Input: part model. Units: mm. Frame: model coordinates. Round coordinates to 2 decimals unless told otherwise and drop trailing zeros. Order: outer loops, then holes, each group sorted by start corner. A loop starts at its lowest first (then second) coordinate and runs counter-clockwise, first axis right, second up. Notation, with made-up numbers: (71.5, 81.5) -> (109.5, 81.5) arc R25 cw to (109.5, 93.5) -> close; hole circle Ø2 at (-19, 79.5). An arc over 180 degrees is marked (long way). Answer as CSV lines item,"result". Start each with the question number.
1) First-contact query: P1, Ø1.4, axis at x = -253.5, z = 2, coming from the +Y side. Flat tip, straight axial feed; report the tip coordinate or a pass-through.
2) Mould query, pull axis Y, two halves, no side actions, for faces 1 (the face through (-220, 38, 0)), 2 (the face through (-4.63, 89.34, 2.35)), 3 (the face through (-208.424, 10.662, 2.348)). Classes: +Y half, -Y half, draft (parallel to the pull), parting line (faces both ways), or undercut.
3) Section query B-B, the plane z = 3.45. State how many separate pieces and enclosed holes the cut face has, and give its area (3 significant figures).
4) Line query: L1, parallel to X at y = 18, z = 1.8; L2, parallel to X at y = 6, z = 0.75; L3, parallel to Y at x = -363, z = 3.3. Output: solid intervals per line, ascending.
5) Section query A-A, the plane y = 4. Output: boundary loops of the cut face in (x, z), and give its area (3 significant figures).
```python
from build123d import *

# Parameters (mm, degrees)
SKETCH1_R           = 14.225
SKETCH1_R_2         = 14.3
SKETCH1_R_3         = 3.18
SKETCH1_R_4         = 1.25
BOSS_EXTRUDE5_DEPTH = 4.7625


with BuildPart() as part:
    # Sketch1 → Boss-Extrude5 (new body)
    with BuildSketch(Plane.XY):
        with BuildLine():
            Line((-438.54516333, 90.490429708), (-13.66516333, 90.490429708))
            ThreePointArc((-13.66516333, 90.490429708), (-4.523203097, 89.26845658), (-0.269770336, 81.084511017))
            Line((-0.269770336, 81.084511017), (-0.269770336, -5.909570292))
            ThreePointArc((-0.269770336, -5.909570292), (-3.198702525, -12.980638104), (-10.269770336, -15.909570292))
            Line((-10.269770336, -15.909570292), (-435.149770336, -15.909570292))
            ThreePointArc((-435.149770336, -15.909570292), (-442.220838148, -12.980638104), (-445.149770336, -5.909570292))
            Line((-445.149770336, -5.909570292), (-445.149770336, 81.084511017))
            ThreePointArc((-445.149770336, 81.084511017), (-443.333715899, 86.831078256), (-438.54516333, 90.490429708))
        make_face()
        with Locations(Location((-394.349770336, 12.790429708, 0), (0, 0, 180))):
            Circle(SKETCH1_R, mode=Mode.SUBTRACT)
        with Locations(Location((-51.069770336, 12.790429708, 0), (0, 0, 180))):
            Circle(SKETCH1_R, mode=Mode.SUBTRACT)
        with Locations(Location((-222.709770336, 11.290429708, 0), (0, 0, 180))):
            Circle(SKETCH1_R_2, mode=Mode.SUBTRACT)
        with Locations(Location((-174.899770336, 13.384511017, 0), (0, 0, 180))):
            Circle(SKETCH1_R_3, mode=Mode.SUBTRACT)
        with Locations(Location((-366.990768764, 12.790429708, 0), (0, 0, 180))):
            Circle(SKETCH1_R_3, mode=Mode.SUBTRACT)
        with Locations(Location((-358.995687615, 21.719099167, 0), (0, 0, 180))):
            Circle(SKETCH1_R_4, mode=Mode.SUBTRACT)
        with Locations(Location((-94.899770336, 13.384511017, 0), (0, 0, 180))):
            Circle(SKETCH1_R_3, mode=Mode.SUBTRACT)
        with Locations(Location((-96.899770336, 21.384511017, 0), (0, 0, 180))):
            Circle(SKETCH1_R_4, mode=Mode.SUBTRACT)
        with Locations(Location((-106.899770336, 21.384511017, 0), (0, 0, 180))):
            Circle(SKETCH1_R_4, mode=Mode.SUBTRACT)
        with Locations(Location((-350.990768764, 12.790429708, 0), (0, 0, 180))):
            Circle(SKETCH1_R_3, mode=Mode.SUBTRACT)
        with Locations(Location((-334.990768764, 12.790429708, 0), (0, 0, 180))):
            Circle(SKETCH1_R_3, mode=Mode.SUBTRACT)
        with Locations(Location((-318.990768764, 12.790429708, 0), (0, 0, 180))):
            Circle(SKETCH1_R_3, mode=Mode.SUBTRACT)
        with Locations(Location((-302.990768764, 12.790429708, 0), (0, 0, 180))):
            Circle(SKETCH1_R_3, mode=Mode.SUBTRACT)
        with Locations(Location((-286.990768764, 12.790429708, 0), (0, 0, 180))):
            Circle(SKETCH1_R_3, mode=Mode.SUBTRACT)
        with Locations(Location((-158.899770336, 13.384511017, 0), (0, 0, 180))):
            Circle(SKETCH1_R_3, mode=Mode.SUBTRACT)
        with Locations(Location((-142.899770336, 13.384511017, 0), (0, 0, 180))):
            Circle(SKETCH1_R_3, mode=Mode.SUBTRACT)
        with Locations(Location((-126.899770336, 13.384511017, 0), (0, 0, 180))):
            Circle(SKETCH1_R_3, mode=Mode.SUBTRACT)
        with Locations(Location((-110.899770336, 13.384511017, 0), (0, 0, 180))):
            Circle(SKETCH1_R_3, mode=Mode.SUBTRACT)
        with Locations(Location((-86.899770336, 21.384511017, 0), (0, 0, 180))):
            Circle(SKETCH1_R_4, mode=Mode.SUBTRACT)
        with Locations(Location((-270.990768764, 12.790429708, 0), (0, 0, 180))):
            Circle(SKETCH1_R_3, mode=Mode.SUBTRACT)
        with Locations(Location((-348.995687615, 21.719099167, 0), (0, 0, 180))):
            Circle(SKETCH1_R_4, mode=Mode.SUBTRACT)
        with Locations(Location((-116.899770336, 21.384511017, 0), (0, 0, 180))):
            Circle(SKETCH1_R_4, mode=Mode.SUBTRACT)
        with Locations(Location((-338.995687615, 21.719099167, 0), (0, 0, 180))):
            Circle(SKETCH1_R_4, mode=Mode.SUBTRACT)
        with Locations(Location((-328.995687615, 21.719099167, 0), (0, 0, 180))):
            Circle(SKETCH1_R_4, mode=Mode.SUBTRACT)
        with Locations(Location((-318.995687615, 21.719099167, 0), (0, 0, 180))):
            Circle(SKETCH1_R_4, mode=Mode.SUBTRACT)
        with Locations(Location((-308.995687615, 21.719099167, 0), (0, 0, 180))):
            Circle(SKETCH1_R_4, mode=Mode.SUBTRACT)
        with Locations(Location((-298.995687615, 21.719099167, 0), (0, 0, 180))):
            Circle(SKETCH1_R_4, mode=Mode.SUBTRACT)
        with Locations(Location((-288.995687615, 21.719099167, 0), (0, 0, 180))):
            Circle(SKETCH1_R_4, mode=Mode.SUBTRACT)
        with Locations(Location((-126.899770336, 21.384511017, 0), (0, 0, 180))):
            Circle(SKETCH1_R_4, mode=Mode.SUBTRACT)
        with Locations(Location((-136.899770336, 21.384511017, 0), (0, 0, 180))):
            Circle(SKETCH1_R_4, mode=Mode.SUBTRACT)
        with Locations(Location((-146.899770336, 21.384511017, 0), (0, 0, 180))):
            Circle(SKETCH1_R_4, mode=Mode.SUBTRACT)
        with Locations(Location((-156.899770336, 21.384511017, 0), (0, 0, 180))):
            Circle(SKETCH1_R_4, mode=Mode.SUBTRACT)
        with Locations(Location((-222.709770336, 85.384511017, 0), (0, 0, 180))):
            Circle(SKETCH1_R_4, mode=Mode.SUBTRACT)
        with Locations(Location((-142.709770336, 78.334511017, 0), (0, 0, 180))):
            Circle(SKETCH1_R_3, mode=Mode.SUBTRACT)
        with Locations(Location((-94.709770336, 78.334511017, 0), (0, 0, 180))):
            Circle(SKETCH1_R_3, mode=Mode.SUBTRACT)
        with Locations(Location((-78.709770336, 78.334511017, 0), (0, 0, 180))):
            Circle(SKETCH1_R_3, mode=Mode.SUBTRACT)
        with Locations(Location((-30.709770336, 78.334511017, 0), (0, 0, 180))):
            Circle(SKETCH1_R_3, mode=Mode.SUBTRACT)
        with Locations(Location((-14.709770336, 78.334511017, 0), (0, 0, 180))):
            Circle(SKETCH1_R_3, mode=Mode.SUBTRACT)
        with Locations(Location((-302.709770336, 78.334511017, 0), (0, 0, 180))):
            Circle(SKETCH1_R_3, mode=Mode.SUBTRACT)
        with Locations(Location((-350.709770336, 78.334511017, 0), (0, 0, 180))):
            Circle(SKETCH1_R_3, mode=Mode.SUBTRACT)
        with Locations(Location((-366.709770336, 78.334511017, 0), (0, 0, 180))):
            Circle(SKETCH1_R_3, mode=Mode.SUBTRACT)
        with Locations(Location((-414.709770336, 78.334511017, 0), (0, 0, 180))):
            Circle(SKETCH1_R_3, mode=Mode.SUBTRACT)
        with Locations(Location((-212.709770336, 85.384511017, 0), (0, 0, 180))):
            Circle(SKETCH1_R_4, mode=Mode.SUBTRACT)
        with Locations(Location((-202.709770336, 85.384511017, 0), (0, 0, 180))):
            Circle(SKETCH1_R_4, mode=Mode.SUBTRACT)
        with Locations(Location((-192.709770336, 85.384511017, 0), (0, 0, 180))):
            Circle(SKETCH1_R_4, mode=Mode.SUBTRACT)
        with Locations(Location((-182.709770336, 85.384511017, 0), (0, 0, 180))):
            Circle(SKETCH1_R_4, mode=Mode.SUBTRACT)
        with Locations(Location((-172.709770336, 85.384511017, 0), (0, 0, 180))):
            Circle(SKETCH1_R_4, mode=Mode.SUBTRACT)
        with Locations(Location((-162.709770336, 85.384511017, 0), (0, 0, 180))):
            Circle(SKETCH1_R_4, mode=Mode.SUBTRACT)
        with Locations(Location((-152.709770336, 85.384511017, 0), (0, 0, 180))):
            Circle(SKETCH1_R_4, mode=Mode.SUBTRACT)
        with Locations(Location((-142.709770336, 85.384511017, 0), (0, 0, 180))):
            Circle(SKETCH1_R_4, mode=Mode.SUBTRACT)
        with Locations(Location((-132.709770336, 85.384511017, 0), (0, 0, 180))):
            Circle(SKETCH1_R_4, mode=Mode.SUBTRACT)
        with Locations(Location((-122.709770336, 85.384511017, 0), (0, 0, 180))):
            Circle(SKETCH1_R_4, mode=Mode.SUBTRACT)
        with Locations(Location((-112.709770336, 85.384511017, 0), (0, 0, 180))):
            Circle(SKETCH1_R_4, mode=Mode.SUBTRACT)
        with Locations(Location((-102.709770336, 85.384511017, 0), (0, 0, 180))):
            Circle(SKETCH1_R_4, mode=Mode.SUBTRACT)
        with Locations(Location((-92.709770336, 85.384511017, 0), (0, 0, 180))):
            Circle(SKETCH1_R_4, mode=Mode.SUBTRACT)
        with Locations(Location((-82.709770336, 85.384511017, 0), (0, 0, 180))):
            Circle(SKETCH1_R_4, mode=Mode.SUBTRACT)
        with Locations(Location((-72.709770336, 85.384511017, 0), (0, 0, 180))):
            Circle(SKETCH1_R_4, mode=Mode.SUBTRACT)
        with Locations(Location((-62.709770336, 85.384511017, 0), (0, 0, 180))):
            Circle(SKETCH1_R_4, mode=Mode.SUBTRACT)
        with Locations(Location((-52.709770336, 85.384511017, 0), (0, 0, 180))):
            Circle(SKETCH1_R_4, mode=Mode.SUBTRACT)
        with Locations(Location((-42.709770336, 85.384511017, 0), (0, 0, 180))):
            Circle(SKETCH1_R_4, mode=Mode.SUBTRACT)
        with Locations(Location((-32.709770336, 85.384511017, 0), (0, 0, 180))):
            Circle(SKETCH1_R_4, mode=Mode.SUBTRACT)
        with Locations(Location((-22.709770336, 85.384511017, 0), (0, 0, 180))):
            Circle(SKETCH1_R_4, mode=Mode.SUBTRACT)
        with Locations(Location((-12.709770336, 85.384511017, 0), (0, 0, 180))):
            Circle(SKETCH1_R_4, mode=Mode.SUBTRACT)
        with Locations(Location((-232.709770336, 85.384511017, 0), (0, 0, 180))):
            Circle(SKETCH1_R_4, mode=Mode.SUBTRACT)
        with Locations(Location((-242.709770336, 85.384511017, 0), (0, 0, 180))):
            Circle(SKETCH1_R_4, mode=Mode.SUBTRACT)
        with Locations(Location((-252.709770336, 85.384511017, 0), (0, 0, 180))):
            Circle(SKETCH1_R_4, mode=Mode.SUBTRACT)
        with Locations(Location((-262.709770336, 85.384511017, 0), (0, 0, 180))):
            Circle(SKETCH1_R_4, mode=Mode.SUBTRACT)
        with Locations(Location((-272.709770336, 85.384511017, 0), (0, 0, 180))):
            Circle(SKETCH1_R_4, mode=Mode.SUBTRACT)
        with Locations(Location((-282.709770336, 85.384511017, 0), (0, 0, 180))):
            Circle(SKETCH1_R_4, mode=Mode.SUBTRACT)
        with Locations(Location((-292.709770336, 85.384511017, 0), (0, 0, 180))):
            Circle(SKETCH1_R_4, mode=Mode.SUBTRACT)
        with Locations(Location((-302.709770336, 85.384511017, 0), (0, 0, 180))):
            Circle(SKETCH1_R_4, mode=Mode.SUBTRACT)
        with Locations(Location((-312.709770336, 85.384511017, 0), (0, 0, 180))):
            Circle(SKETCH1_R_4, mode=Mode.SUBTRACT)
        with Locations(Location((-322.709770336, 85.384511017, 0), (0, 0, 180))):
            Circle(SKETCH1_R_4, mode=Mode.SUBTRACT)
        with Locations(Location((-332.709770336, 85.384511017, 0), (0, 0, 180))):
            Circle(SKETCH1_R_4, mode=Mode.SUBTRACT)
        with Locations(Location((-342.709770336, 85.384511017, 0), (0, 0, 180))):
            Circle(SKETCH1_R_4, mode=Mode.SUBTRACT)
        with Locations(Location((-352.709770336, 85.384511017, 0), (0, 0, 180))):
            Circle(SKETCH1_R_4, mode=Mode.SUBTRACT)
        with Locations(Location((-362.709770336, 85.384511017, 0), (0, 0, 180))):
            Circle(SKETCH1_R_4, mode=Mode.SUBTRACT)
        with Locations(Location((-372.709770336, 85.384511017, 0), (0, 0, 180))):
            Circle(SKETCH1_R_4, mode=Mode.SUBTRACT)
        with Locations(Location((-382.709770336, 85.384511017, 0), (0, 0, 180))):
            Circle(SKETCH1_R_4, mode=Mode.SUBTRACT)
        with Locations(Location((-392.709770336, 85.384511017, 0), (0, 0, 180))):
            Circle(SKETCH1_R_4, mode=Mode.SUBTRACT)
        with Locations(Location((-402.709770336, 85.384511017, 0), (0, 0, 180))):
            Circle(SKETCH1_R_4, mode=Mode.SUBTRACT)
        with Locations(Location((-412.709770336, 85.384511017, 0), (0, 0, 180))):
            Circle(SKETCH1_R_4, mode=Mode.SUBTRACT)
        with Locations(Location((-422.709770336, 85.384511017, 0), (0, 0, 180))):
            Circle(SKETCH1_R_4, mode=Mode.SUBTRACT)
        with Locations(Location((-432.709770336, 85.384511017, 0), (0, 0, 180))):
            Circle(SKETCH1_R_4, mode=Mode.SUBTRACT)
        with Locations(Location((-430.709770336, 78.334511017, 0), (0, 0, 180))):
            Circle(SKETCH1_R_3, mode=Mode.SUBTRACT)
        with Locations(Location((-230.709770336, 78.334511017, 0), (0, 0, 180))):
            Circle(SKETCH1_R_3, mode=Mode.SUBTRACT)
        with Locations(Location((-214.709770336, 78.334511017, 0), (0, 0, 180))):
            Circle(SKETCH1_R_3, mode=Mode.SUBTRACT)
        with Locations(Location((-398.709770336, 78.334511017, 0), (0, 0, 180))):
            Circle(SKETCH1_R_3, mode=Mode.SUBTRACT)
        with Locations(Location((-382.709770336, 78.334511017, 0), (0, 0, 180))):
            Circle(SKETCH1_R_3, mode=Mode.SUBTRACT)
        with Locations(Location((-46.709770336, 78.334511017, 0), (0, 0, 180))):
            Circle(SKETCH1_R_3, mode=Mode.SUBTRACT)
        with Locations(Location((-62.709770336, 78.334511017, 0), (0, 0, 180))):
            Circle(SKETCH1_R_3, mode=Mode.SUBTRACT)
    extrude(amount=BOSS_EXTRUDE5_DEPTH)


solid = part.part
```
Findings:
1,P1,"stops at y = 90.49"
2,face 1,"draft"
2,face 2,"+Y half"
2,face 3,"undercut"
3,separate pieces,"1"
3,enclosed holes,"91"
3,area,"44,100 mm^2"
4,L1,"x = -445.15 to -407.59, -381.11 to -235.34, -210.08 to -64.31, -37.83 to -0.27"
4,L2,"x = -445.15 to -406.85, -381.85 to -236, -209.42 to -63.57, -38.57 to -0.27"
4,L3,"y = -15.91 to 84.17, 86.6 to 90.49"
5,outline,"(-445.15, 0) -> (-405.53, 0) -> (-405.53, 4.76) -> (-445.15, 4.76) -> close; (-383.17, 0) -> (-235.01, 0) -> (-235.01, 4.76) -> (-383.17, 4.76) -> close; (-210.41, 0) -> (-62.25, 0) -> (-62.25, 4.76) -> (-210.41, 4.76) -> close; (-39.89, 0) -> (-0.27, 0) -> (-0.27, 4.76) -> (-39.89, 4.76) -> close"
5,area,"1,790 mm^2"
